Could you check a few things on this model? Use its own coordinates, in mm. Face numbers are marked on the shaded views. A direction names the side the tool comes from. Coordinates: 2 decimals unless noted, no trailing zeros. Loops run counter-clockwise (first coordinate to the right, second up) from the corner with the lowest first, then second, coordinate; pieces in that order, holes last. Notation, with made-up numbers: (57.5, 81.25) -> (105.5, 81.25) arc R33 ccw to (105.5, 109.25) -> close; hole circle Ø2 at (-34.5, 22). An arc over 180 degrees is marked (long way). One line per question, with ' | ' between items.
from build123d import *

# Parameters (mm, degrees)
F1_DEPTH = 20
F2_R     = 2.2
F3_DEPTH = 25


with BuildPart() as f1:
    # F0 (on Top) → F1 (new body)
    with BuildSketch(Plane.XY):
        with BuildLine():
            Line((18.46081, 10.690042), (-25.588245, 10.690042))
            Line((-25.588245, 10.690042), (-25.588245, 4.606251))
            Line((-25.588245, 4.606251), (-12.993412, 4.606251))
            Line((-12.993412, 4.606251), (-12.993412, -7.821557))
            ThreePointArc((-12.993412, -7.821557), (-11.987899, -10.828894), (-9.375783, -12.626664))
            Line((-9.375783, -12.626664), (-9.375783, -14.446242))
            Line((-9.375783, -14.446242), (-4.726099, -14.446242))
            Line((-4.726099, -14.446242), (-4.726099, -11.10937))
            ThreePointArc((-4.726099, -11.10937), (-3.428711, 0.77544), (-2.667342, -11.155706))
            Line((-2.667342, -11.155706), (-2.69909, -14.446242))
            Line((-2.69909, -14.446242), (2.101209, -14.492556))
            Line((2.101209, -14.492556), (2.101209, -12.726463))
            ThreePointArc((2.101209, -12.726463), (4.587048, -10.908086), (5.535637, -7.977886))
            Line((5.535637, -7.977886), (5.535637, 4.606251))
            Line((5.535637, 4.606251), (18.46081, 4.606251))
            Line((18.46081, 4.606251), (18.46081, 10.690042))
        make_face()
    extrude(amount=F1_DEPTH)

    # F2 (on face) → F3 (cut)
    with BuildSketch(Plane(origin=(0, 10.690042, 0), x_dir=(-1, 0, 0), z_dir=(0, 1, 0))):
        with Locations((-12.580651, 10)):
            Circle(F2_R)
        with Locations((19.604826, 10)):
            Circle(F2_R)
    extrude(amount=-F3_DEPTH, mode=Mode.SUBTRACT)


solid = f1.part
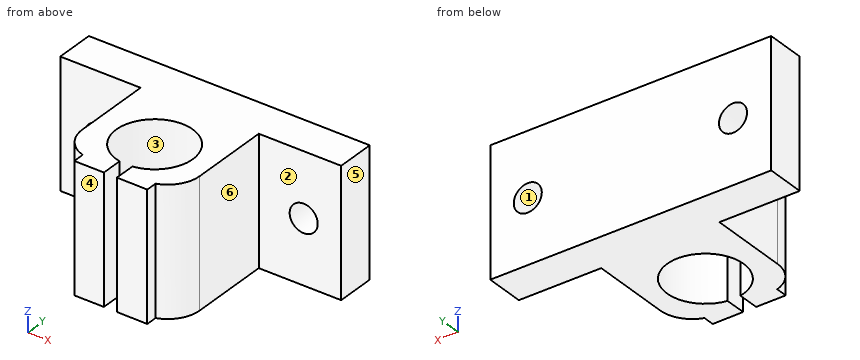
1) I need wall thicknesses on line 1 along X through (y, z) = (3.25, 5.25); line 2 along Y through (x, z) = (14, 4.5); line 3 along X through (y, z) = (-3.25, 19). Which ranges of each line are inside material? Lowest first, please. Write a range as from..to.
Data:
line 1: -12.99..5.54 | line 2: 4.61..10.69 | line 3: -12.99..-9.23, 2.1..5.54
2) If we section it at D-D on z = 3: Please give me the cut outline in (x, y).
Data:
outline: (-25.59, 4.61) -> (-12.99, 4.61) -> (-12.99, -7.82) arc R5 ccw to (-9.38, -12.63) -> (-9.38, -14.45) -> (-4.73, -14.45) -> (-4.73, -11.11) arc R6 cw (long way) to (-2.67, -11.16) -> (-2.7, -14.45) -> (2.1, -14.49) -> (2.1, -12.73) arc R5 ccw to (5.54, -7.98) -> (5.54, 4.61) -> (18.46, 4.61) -> (18.46, 10.69) -> (-25.59, 10.69) -> close
3) On a 3-axis mill with a long thin cutter (end or side, diameter ignored), from which of +Z, -Z, +X, -X, +Y, -Y can I reach the whole of each face in a straight line? I mean the marked faces 4, 5 and 6. Say none if no direction works.
Data:
face 4: +Z, -Z, -X, -Y | face 5: +Z, -Z, +X, +Y, -Y | face 6: +Z, -Z, +X, -Y
4) I'm going to push flat-ended pins straight in: pin 1 Ø3.5 at (y, z) = (-13, 5.5) entering from +X; pin 2 Ø8 at (x, z) = (-4, 11) entering from -Y; pin 3 Ø0.5 at (y, z) = (-13.5, 15) entering from -X. Where does each tip first touch, or does it pass through?
Data:
pin 1: x = 4.32 | pin 2: y = -14.47 | pin 3: x = -9.38
5) If we section it at C-C on y = -2.75: Please give me the cut outline in (x, z).
Data:
outline: (-12.99, 0) -> (-9.03, 0) -> (-9.03, 20) -> (-12.99, 20) -> close; (1.9, 0) -> (5.54, 0) -> (5.54, 20) -> (1.9, 20) -> close
6) If we section it at A-A on z = 10: Please give me the cut outline in (x, y).
Data:
outline: (-25.59, 4.61) -> (-21.8, 4.61) -> (-21.8, 10.69) -> (-25.59, 10.69) -> close; (-17.4, 4.61) -> (-12.99, 4.61) -> (-12.99, -7.82) arc R5 ccw to (-9.38, -12.63) -> (-9.38, -14.45) -> (-4.73, -14.45) -> (-4.73, -11.11) arc R6 cw (long way) to (-2.67, -11.16) -> (-2.7, -14.45) -> (2.1, -14.49) -> (2.1, -12.73) arc R5 ccw to (5.54, -7.98) -> (5.54, 4.61) -> (10.38, 4.61) -> (10.38, 10.69) -> (-17.4, 10.69) -> close; (14.78, 4.61) -> (18.46, 4.61) -> (18.46, 10.69) -> (14.78, 10.69) -> close
7) If we section it at B-B on x = 0: Please give me the cut outline in (y, z), and give its area (3 significant figures).
Data:
outline: (-14.47, 0) -> (-10.05, 0) -> (-10.05, 20) -> (-14.47, 20) -> close; (-0.4, 0) -> (10.69, 0) -> (10.69, 20) -> (-0.4, 20) -> close | area: 310 mm²
8) We'd pull the mould along Y, two halves only. Please class the marked faces 1, 2 and 3: pulls with the +Y half, pulls with the -Y half, needs draft (parallel to the pull), parting line crosses it, or undercut.
Data:
face 1: needs draft | face 2: pulls with the -Y half | face 3: undercut
